from build123d import *

# Parameters (mm, degrees)
F0_W     = 42
F0_H     = 20
F1_DEPTH = 25


with BuildPart() as f1:
    # F0 (on Front) → F1 (new body)
    with BuildSketch(Plane.XZ):
        Polygon((0, -45), (0, 0), (-43, 0), (-45, 0), (-45, -45), align=None)
        Polygon((-43, 0), (0, 0), (0, 3), (-42, 3), (-43, 3), align=None)
        with Locations((-21, 13)):
            Rectangle(F0_W, F0_H)
        Polygon((0, -53), (0, -45), (-45, -45), (-48, -45), (-48, -53), align=None)
    extrude(amount=F1_DEPTH)


solid = f1.part
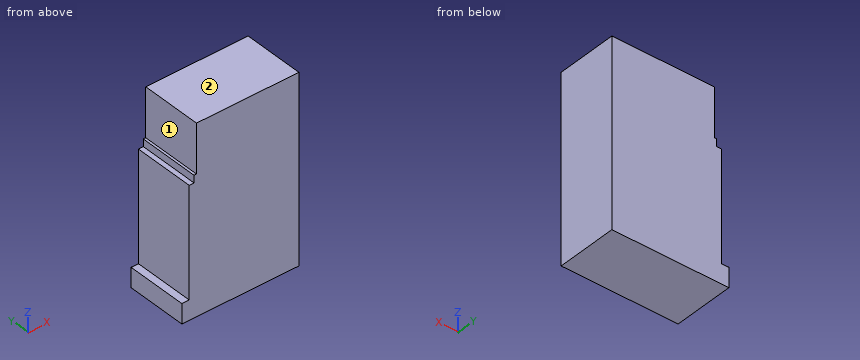
CAD build for the part. Positions are in the model's coordinates, mm. Face numbers are marked on the shaded views. A direction names the side the tool comes from. Coordinates: 2 decimals unless noted, no trailing zeros. Write each loop counter-clockwise with the first axis right and the second up, starting at its lowest first coordinate (ties: lowest second). Pieces come first, ordered by that corner, then holes. Notation, with made-up numbers: M 2,-4.5 L 56,-4.5 A35 ccw 56,29.5 Z; hole C 37,41 d7. An arc over 180 degrees is marked long. Answer as a JSON object with one key per item and string values. Group by question number.
1) Wall check: line 1 (X direction, y = -23.5, z = -38); line 2 (X direction, y = -1.75, z = 9.5). Give the ranges that are in metal, low to high. Write a range as from..to.
2) Saw through at B-B (z = -20.5). Write the cut outline in (x, y).
3) Tool access for the marked faces 1 and 2: list every direction of +Z, -Z, +X, -X, +Y, -Y with a clear straight run to the whole face (end or side of a thin tool).
4) Saw through at A-A (y = -13.25). Write the cut outline in (x, z).
5) Saw through at C-C (x = -44). Write the cut outline in (y, z), plus the area to 4 significant figures.
6) Pin check, flat tips, straight feed: pin 1 Ø12 at (y, z) = (-17, 2) entering from +X; pin 2 Ø10 at (y, z) = (-18.5, 15) entering from -X; pin 3 Ø2.5 at (x, y) = (-47, -17) entering from +Z; pin 4 Ø1.6 at (x, y) = (-44.5, -18) entering from +Z. Stop position of each tip, or through.
Values follow:
{
 "1": {"line 1": "x = -45..0", "line 2": "x = -42..0"},
 "2": {"outline": "M -45,-25 L 0,-25 L 0,0 L -45,0 Z"},
 "3": {"face 1": "+Z, -X, +Y, -Y", "face 2": "+Z, +X, -X, +Y, -Y"},
 "4": {"outline": "M -48,-53 L 0,-53 L 0,23 L -42,23 L -42,3 L -43,3 L -43,0 L -45,0 L -45,-45 L -48,-45 Z"},
 "5": {"outline": "M -25,-53 L 0,-53 L 0,0 L -25,0 Z", "area": "1,325 mm2"},
 "6": {"pin 1": "stops at x = 0", "pin 2": "stops at x = -42", "pin 3": "stops at z = -45", "pin 4": "stops at z = 0"}
}
